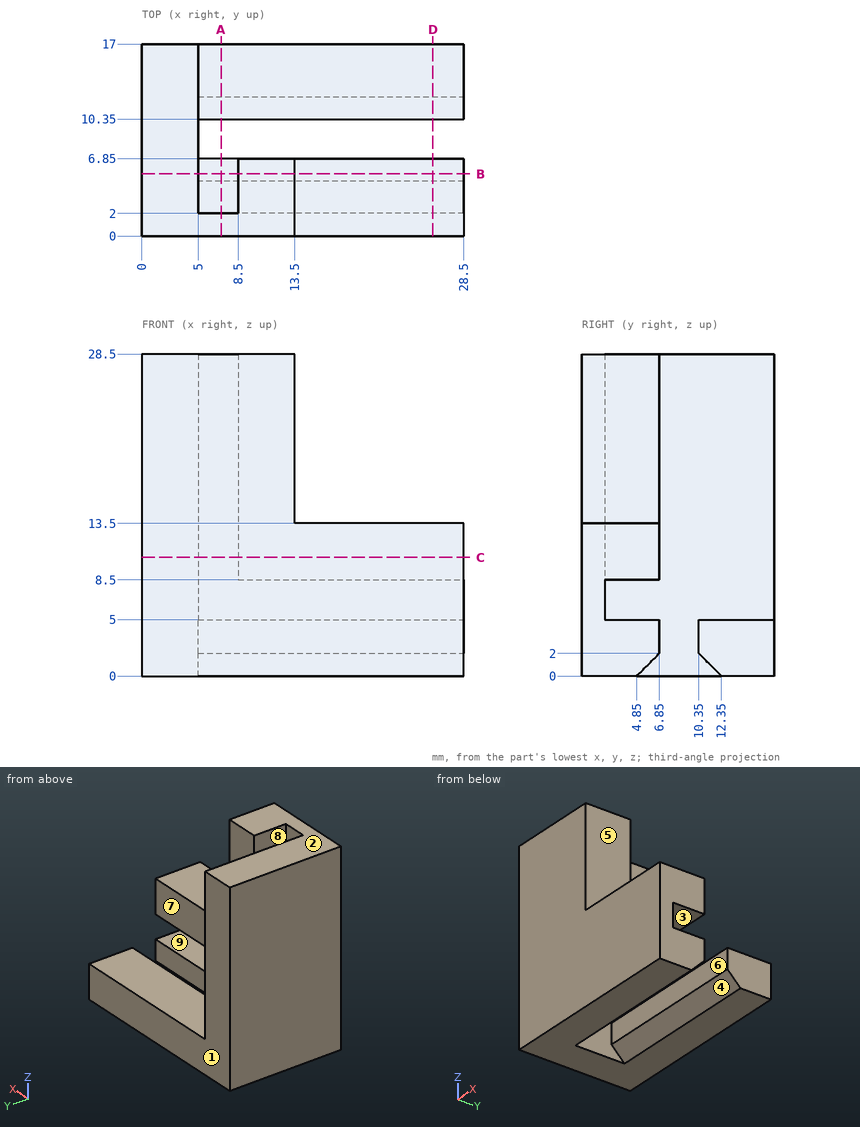
Verification items for this drawing (mm, ordinates from the low corner). A direction names the side the tool comes from. Round coordinates to 2 decimals unless told otherwise and drop trailing zeros. Write each loop counter-clockwise with the first axis right and the second up, starting at its lowest first coordinate (ties: lowest second). Pieces come first, ordered by that corner, then holes. Notation, with made-up numbers: M 25,-29.5 L 60,-29.5 A26 cw 60,-3.5 Z; hole C 52.5,-1.5 d10. An arc over 180 degrees is marked long. Write item = value, one per line. Start each with the question number.
1. Release check for a two-part mould opening along Z. For the marked faces 1, 2, 3 and 4 record: pulls with the +Z half, pulls with the -Z half, needs draft (parallel to the pull), parting line crosses it, or undercut.
2. Section check B-B, the plane y = 5.5. Record the cut outline in (x, z).
3. Gauge pin test, flat ends, axial feed: pin 1 (2 mm diameter, centred on x = 14.5, y = 12, fed in from -Z); pin 2 (1.5 mm diameter, centred on x = 16.5, y = 5.5, fed in from +Z); pin 3 (10 mm diameter, centred on x = 16, z = 19.5, fed in from +Y); pin 4 (1 mm diameter, centred on y = 14, z = 8.5, fed in from +X). Record the tip position at first contact, or that the pin passes through.
4. Section check D-D, the plane x = 25.75. Record the cut outline in (y, z).
5. Section check A-A, the plane x = 7. Record the cut outline in (y, z), then the cut area to 4 significant figures.
6. Scan lines: line 1 (Z direction, x = 25.5, y = 2.75); line 2 (Z direction, x = 9, y = 3.5). Record each from-to range of solid material in increasing order. Write a range as [from, to].
7. Tool access check on the marked faces 5, 6, 7, 8 and 9. Record the directions out of +Z, -Z, +X, -X, +Y, -Y that give a thin tool (end or side, any length) a straight path to the whole face; none if there is none.
8. Section check C-C, the plane z = 10.5. Record the cut outline in (x, y), then the cut area to 3 significant figures.
Results found:
q1.face_1 = needs draft
q1.face_2 = pulls with the +Z half
q1.face_3 = undercut
q1.face_4 = pulls with the -Z half
q2.outline = M 0,0 L 5,0 L 5,0.65 L 28.5,0.65 L 28.5,5 L 5,5 L 5,28.5 L 0,28.5 Z; M 8.5,8.5 L 28.5,8.5 L 28.5,13.5 L 13.5,13.5 L 13.5,28.5 L 8.5,28.5 Z
q3.pin_1 = 0
q3.pin_2 = 13.5
q3.pin_3 = 6.85
q3.pin_4 = 5
q4.outline = M 0,0 L 4.85,0 L 6.85,2 L 6.85,5 L 2,5 L 2,8.5 L 6.85,8.5 L 6.85,13.5 L 0,13.5 Z; M 10.35,2 L 12.35,0 L 17,0 L 17,5 L 10.35,5 Z
q5.outline = M 0,0 L 4.85,0 L 6.85,2 L 6.85,5 L 2,5 L 2,28.5 L 0,28.5 Z; M 10.35,2 L 12.35,0 L 17,0 L 17,5 L 10.35,5 Z
q5.area = 110.5 mm^2
q6.line_1 = [0, 5], [8.5, 13.5]
q6.line_2 = [0, 5], [8.5, 28.5]
q7.face_5 = +Z, +X, +Y, -Y
q7.face_6 = +Z, -Z, +X
q7.face_7 = +Z, -Z, +X, +Y
q7.face_8 = +Z, +Y
q7.face_9 = +X, +Y
q8.outline = M 0,0 L 28.5,0 L 28.5,6.85 L 8.5,6.85 L 8.5,2 L 5,2 L 5,17 L 0,17 Z
q8.area = 229 mm^2
